Autodesk Inventor part; units mm, degrees
ref_plane "YZ Plane" through (0, 0, 0) normal (1, 0, 0) x (0, 1, 0)
ref_plane "XZ Plane" through (0, 0, 0) normal (0, 1, 0) x (-1, 0, 0)
ref_plane "XY Plane" through (0, 0, 0) normal (0, 0, 1) x (1, 0, 0)
sketch "Sketch1" plane through (0, 0, 0) normal (0, 1, 0) x (-1, 0, 0)
  arc A0 (6.1484, 1.5875) -> (6.1484, -1.5875) centre (0, 0) ccw
  line L0 (6.1484, 1.5875) -> (4.5604, 1.5875)
  line L1 (4.5604, 1.5875) -> (4.5604, -1.5875)
  line L2 (4.5604, -1.5875) -> (6.1484, -1.5875)
  line L3 (4.5604, 0) -> (0, 0) construction
  dimension "d0" = 12.7
  dimension "d1" = 3.175
  dimension "d2" = 1.588
extrude "Extrusion1" add sketch "Sketch1" along normal blind 95.25
chamfer "Chamfer1" distance 1 angle 45 2 edges at (6.35, 0, 0) (6.35, 95.25, 0)
hole "Hole1" at (0, 0, 0) direction (0, 1, 0) diameter 4.2 depth 14 tip angle 118
hole "Hole2" at (0, 95.25, 0) direction (0, -1, 0) diameter 4.2 depth 14 tip angle 118
sketch "Sketch2" plane through (0, 0, 0) normal (0, 0, 1) x (1, 0, 0)
  line L0 (0, 0) -> (0, 95.25) construction
  line L1 (-2.1, 95.25) -> (2.1, 95.25) construction
  line L2 (-6.35, 14.775) -> (-6.0452, 14.775)
  line L3 (-6.0452, 14.775) -> (-6.0452, 15.875)
  line L4 (-6.0452, 15.875) -> (-6.35, 15.875)
  line L5 (-6.35, 15.875) -> (-6.35, 14.775)
  dimension "d30" = 1.1
  dimension "d32" = 6.35
  dimension "d33" = 79.375
  dimension "d38" = 6.0452
revolve "Revolution1" cut sketch "Sketch2" angle 360 about axis through (0, 0, 0) along (0, 1, 0)
properties part number "Drum_Axle" material "Steel, High Strength, Low Alloy"
Verification items for the finished model (mm, model axes). A direction names the side the tool comes from. Round coordinates to 2 decimals unless told otherwise and drop trailing zeros. Write each loop counter-clockwise with the first axis right and the second up, starting at its lowest first coordinate (ties: lowest second). Pieces come first, ordered by that corner, then holes. Notation, with made-up numbers: (28.25, 7.5) -> (69.25, 7.5) arc R16 ccw to (69.25, 24.5) -> close; hole circle Ø2 at (6, 13.25). An arc over 180 degrees is marked (long way). Write each question's results on one line, items separated by ' | '. Start each with the question number.
1. Material ranges on probe 1 along X at (y, z) = (85, 0); probe 2 along Z at (x, y) = (0, 84.75); probe 3 along Z at (x, y) = (-5, 19), recorded low to high. Write a range as from..to.
2. Set-up check for faces 1 (the cylindrical face through (-0.631, 88.152, 2.003)), 2 (the flat face through (-5, 47, -1.588)), 3 (the cylindrical face through (-0.631, 7.098, -2.003)): record each of +Z, -Z, +X, -X, +Y, -Y from which the full face is reachable in a straight line by a thin tool's end or side.
3. Draft check along Y on faces 4 (the flat face through (0.2, 0, -2.3)), 5 (the flat face through (0.2, 95.25, -2.3)), 6 (the cylindrical face through (6.04, 15.33, 0.24)). Enter one of: +Y half, -Y half, draft (parallel to the pull), parting line (faces both ways), or undercut.
4. Depth check by flat-ended pin: P1, Ø6, axis at x = 5, z = -0.5, coming from the -Y side; P2, Ø1.3, axis at x = -5.5, y = 53, coming from the -Z side; P3, Ø1, axis at y = 41, z = -2, coming from the +X side; P4, Ø0.8, axis at x = -5.5, y = 46, coming from the +Z side. Enter the tip coordinate at first touch or a pass-through.
5. Cross-section at B-B (y = 66.5). Enter the section's corners in (x, z), then the cut area to 3 significant figures.
6. Cross-section at A-A (y = 12). Enter the section's corners in (x, z), then the cut area to 3 significant figures.
Solutions:
1) probe 1: x = -4.56..-2.1, 2.1..6.35 | probe 2: z = -6.35..-2.1, 2.1..6.35 | probe 3: z = -3.91..-1.59, 1.59..3.91
2) face 1: +Y | face 2: -X, +Y, -Y | face 3: -Y
3) face 4: -Y half | face 5: +Y half | face 6: undercut
4) P1: stops at y = 0 | P2: stops at z = -4.1 | P3: stops at x = 6.17 | P4: stops at z = 3.78
5) outline: (-6.15, -1.59) arc R6.35 ccw (long way) to (-6.15, 1.59) -> (-4.56, 1.59) -> (-4.56, -1.59) -> close | area: 121 mm2
6) outline: (-6.15, -1.59) arc R6.35 ccw (long way) to (-6.15, 1.59) -> (-4.56, 1.59) -> (-4.56, -1.59) -> close; hole circle Ø4.2 at (0, 0) | area: 107 mm2
